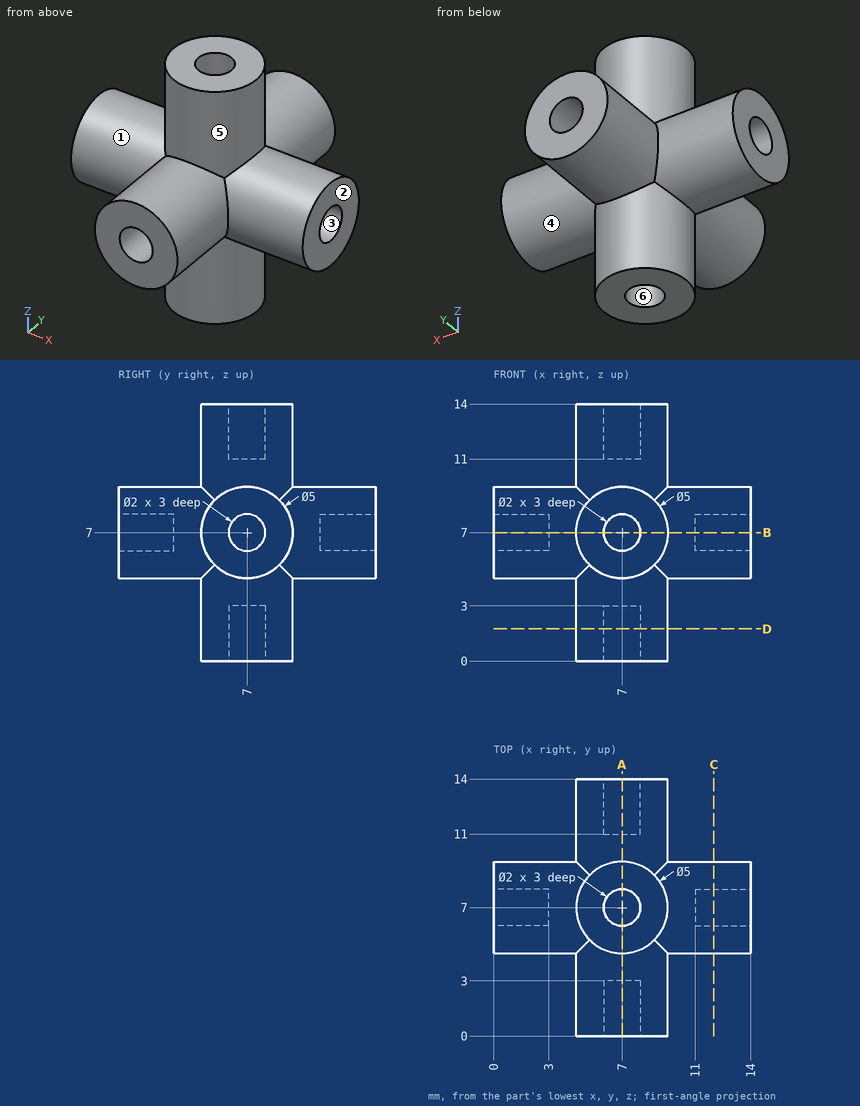
Study the drawing (mm; zero at the part's minimum x, y, z) and answer. A direction names the side the tool comes from. Give positions to 0.01 mm unless a question says otherwise; leave off trailing zeros. Write each loop counter-clockwise with the first axis right and the second up, starting at its lowest first coordinate (ties: lowest second). Pieces come first, ordered by that corner, then holes. Notation, with made-up numbers: M -10.75,-7 L 4.25,-7 A34 cw 4.25,27 Z; hole C 3.5,87.5 d3. An arc over 180 degrees is marked long. Put each result on its own line as item: value. Start each with the question number.
1. For a pull along Y with two mould halves and no side action, classify the marked faces 1, 2 and 3 as released by +Y, released by -Y, zero draft, split by the parting line, or undercut.
2. Each of these flat-tipped pins is pushed along its axis until it touches: pin 1 Ø0.6 at (x, z) = (7, 7) entering from -Y; pin 2 Ø4 at (x, y) = (12.5, 9) entering from -Z; pin 3 Ø2 at (y, z) = (3.5, 6) entering from -X. Where does it stop, or does it pass through?
3. The part is cut by section A-A, the plane x = 7. Give the vertices of the cut face in (y, z).
4. The part is cut by section C-C, the plane x = 12. Give the vertices of the cut face in (y, z), and give its area (3 significant figures).
5. Consider line 1 along Z through (x, y) = (7, 12.05). Determine where the line is inside the solid, lowest interval first.
6. Which of the six approach directions +Z, -Z, +X, -X, +Y, -Y give full straight-line access (tool end or side, diameter ignored) to the marked faces 4, 5 and 6?
Final values:
1. face 1: split by the parting line
1. face 2: zero draft
1. face 3: undercut
2. pin 1: stops at y = 3
2. pin 2: stops at z = 4.5
2. pin 3: stops at x = 4.5
3. outline: M 0,4.5 L 4.5,4.5 L 4.5,0 L 6,0 L 6,3 L 8,3 L 8,0 L 9.5,0 L 9.5,4.5 L 14,4.5 L 14,6 L 11,6 L 11,8 L 14,8 L 14,9.5 L 9.5,9.5 L 9.5,14 L 8,14 L 8,11 L 6,11 L 6,14 L 4.5,14 L 4.5,9.5 L 0,9.5 L 0,8 L 3,8 L 3,6 L 0,6 Z
4. outline: C 7,7 d5; hole C 7,7 d2
4. area: 16.5 mm²
5. line 1: z = 4.5 to 6, 8 to 9.5
6. face 4: +X
6. face 5: +Z
6. face 6: -Z
